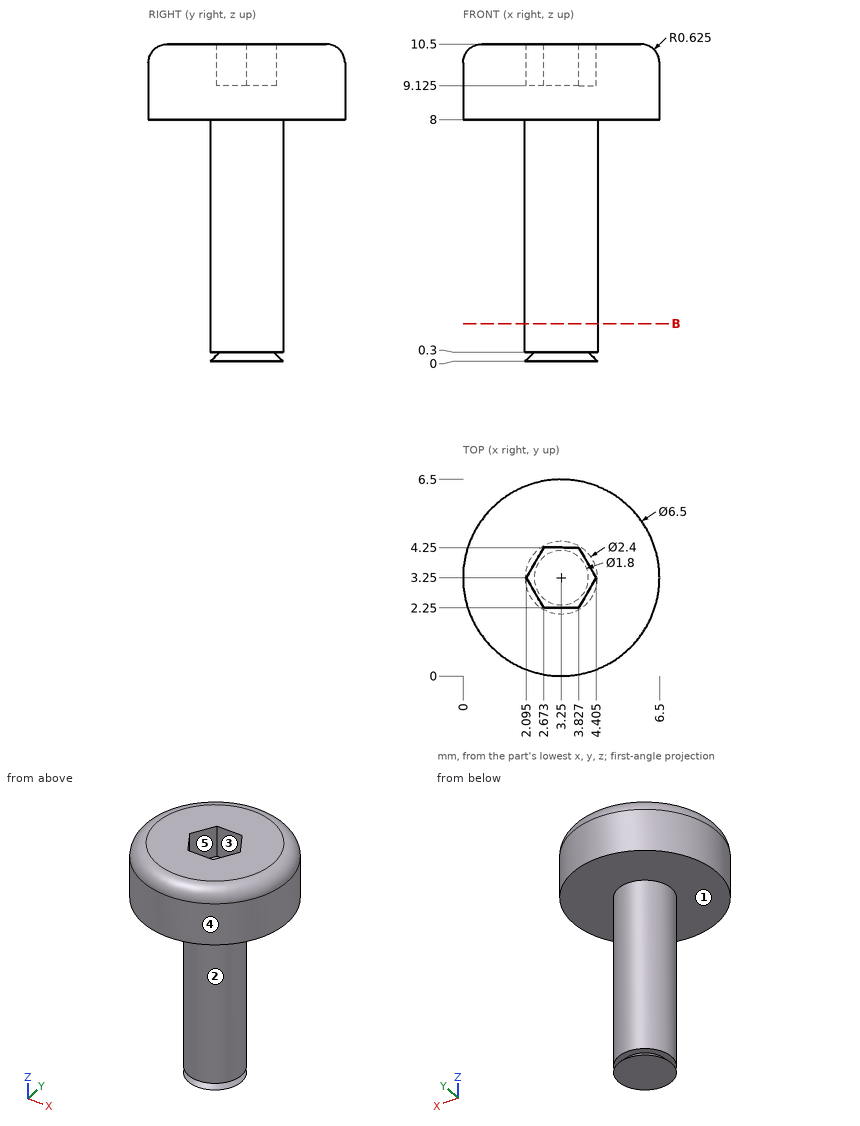
Study the drawing (mm; zero at the part's minimum x, y, z) and answer. A direction names the side the tool comes from. Give positions to 0.01 mm unless a question says otherwise; leave off trailing zeros. Write each loop counter-clockwise with the first axis right and the second up, starting at its lowest first coordinate (ties: lowest second). Pieces come first, ordered by that corner, then holes. Notation, with made-up numbers: (7, 44.5) -> (50, 44.5) arc R22 cw to (50, 60.5) -> close; hole circle Ø9 at (22.5, 27.25). An arc over 180 degrees is marked (long way). Write item = value, one per line. Start each with the question number.
1) The part is cut by section B-B, the plane z = 1.25. Determine the outline of the cut face in (x, y).
2) Each of these flat-tipped pins is pushed along its axis until it touches: pin 1 (1 mm diameter, centred on x = 5.5, y = 4.5, fed in from -Z); pin 2 (1.5 mm diameter, centred on y = 2, z = 1.5, fed in from -X); pin 3 (1.5 mm diameter, centred on y = 5, z = 6.5, fed in from +X) (1 decimal). Where does it stop, or does it pass through?
3) Which of the six approach directions +Z, -Z, +X, -X, +Y, -Y give full straight-line access (tool end or side, diameter ignored) to the marked faces 4 and 5?
4) Straight lines are drawn through the part: line 1 along Z through (x, y) = (3.25, 5.25); line 2 along Y through (x, z) = (1.25, 9); line 3 along X through (y, z) = (4, 7.25) (1 decimal). For each, find the intervals that lie inside material, in ascending order.
5) Determine the mould class of the marked faces 1, 2 and 3 for opening direction Y: +Y half, -Y half, draft (parallel to the pull), parting line (faces both ways), or undercut.
Solutions:
q1.outline = circle Ø2.4 at (3.25, 3.25)
q2.pin_1 = 8
q2.pin_2 = 2.16
q2.pin_3 = 3.9
q3.face_4 = +Z, -Z
q3.face_5 = +Z
q4.line_1 = 8 to 10.5
q4.line_2 = 0.69 to 5.81
q4.line_3 = 2.3 to 4.2
q5.face_1 = draft
q5.face_2 = parting line
q5.face_3 = undercut
